```python
from build123d import *

# Parameters (mm, degrees)
F0_R     = 38.1
F0_R_2   = 31.750001
F1_DEPTH = 104.775
F2_R     = 2.4892
F3_DEPTH = 101.6
F4_R     = 2.4892
F5_DEPTH = 101.6


with BuildPart() as f1:
    # F0 (on Front) → F1 (new body, symmetric)
    with BuildSketch(Plane.XZ):
        Circle(F0_R)
        Circle(F0_R_2, mode=Mode.SUBTRACT)
    extrude(amount=F1_DEPTH, both=True)

    # F2 (on Right) → F3 (cut, symmetric)
    with BuildSketch(Plane.YZ):
        with Locations((95.25, 0)):
            Circle(F2_R)
        with Locations((-95.25, 0)):
            Circle(F2_R)
    extrude(amount=F3_DEPTH, both=True, mode=Mode.SUBTRACT)

    # F4 (on Top) → F5 (cut, symmetric)
    with BuildSketch(Plane.XY):
        with Locations((0, 95.25)):
            Circle(F4_R)
        with Locations((0, -95.25)):
            Circle(F4_R)
    extrude(amount=F5_DEPTH, both=True, mode=Mode.SUBTRACT)


solid = f1.part
```
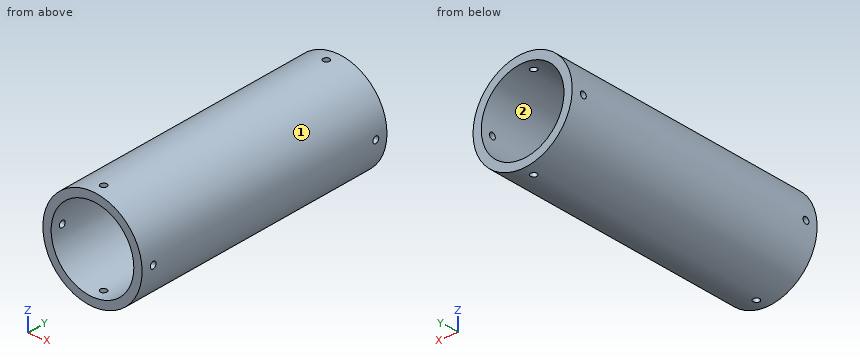
Geometry check sheet. Reference: the model listing, model coordinates, mm. Face numbers are marked on the shaded views. Coordinates: 2 decimals unless noted, no trailing zeros. Write each loop counter-clockwise with the first axis right and the second up, starting at its lowest first coordinate (ties: lowest second). Pieces come first, ordered by that corner, then holes. Notation, with made-up numbers: M 31,-17 L 53,-17 A26 cw 53,14 Z; hole C 86.25,69.25 d6. An arc over 180 degrees is marked long. One line per item, written item: value. Start each with the question number.
(1) Sectioned sample at D-D, the plane z = 16. Enter the section's corners in (x, y) (3 decimals), and give its area (3 significant figures).
(2) Sectioned sample at A-A, the plane x = 0. Enter the section's corners in (y, z) (3 decimals), and give its area (3 significant figures).
(3) Depth check by flat-ended pin: pin 1 (6 mm diameter, centred on y = 34.5, z = -18, fed in from +X); pin 2 (12 mm diameter, centred on x = 8.5, y = -66.5, fed in from -Z); pin 3 (1.5 mm diameter, centred on y = -42.5, z = -16, fed in from -X); pin 4 (1 mm diameter, centred on x = -27.5, z = -10, fed in from -Y). Enter the tip coordinate at first touch or a pass-through.
(4) Sectioned sample at B-B, the plane z = 0. Enter the section's corners in (x, y) (3 decimals), and give its area (3 significant figures).
(5) Scan lines: line 1 along Y through (x, z) = (0, -34.25) (3 decimals); line 2 along Z through (x, y) = (-0.5, 21); line 3 along Z through (x, y) = (-33, -95). Record each from-to range of solid material in increasing order. Write a range as [from, to].
(6) Sectioned sample at C-C, the plane y = -95.25. Enter the section's corners in (x, z), and give its area (3 significant figures).
(7) Release check for a two-part mould opening along Z. For the marked faces 1 and 2 record: released by +Z, released by -Z, zero draft, split by the parting line, or undercut.
Filled sheet:
1. outline: M -34.578,-104.775 L -27.424,-104.775 L -27.424,104.775 L -34.578,104.775 Z; M 27.424,-104.775 L 34.578,-104.775 L 34.578,104.775 L 27.424,104.775 Z
1. area: 3,000 mm²
2. outline: M -104.775,-38.1 L -97.739,-38.1 L -97.739,-31.75 L -104.775,-31.75 Z; M -104.775,31.75 L -97.739,31.75 L -97.739,38.1 L -104.775,38.1 Z; M -92.761,-38.1 L 92.761,-38.1 L 92.761,-31.75 L -92.761,-31.75 Z; M -92.761,31.75 L 92.761,31.75 L 92.761,38.1 L -92.761,38.1 Z; M 97.739,-38.1 L 104.775,-38.1 L 104.775,-31.75 L 97.739,-31.75 Z; M 97.739,31.75 L 104.775,31.75 L 104.775,38.1 L 97.739,38.1 Z
2. area: 2,530 mm²
3. pin 1: x = 35.02
3. pin 2: z = -38.02
3. pin 3: x = -34.91
3. pin 4: through
4. outline: M -38.1,-104.775 L -31.75,-104.775 L -31.75,-97.739 L -38.1,-97.739 Z; M -38.1,-92.761 L -31.75,-92.761 L -31.75,92.761 L -38.1,92.761 Z; M -38.1,97.739 L -31.75,97.739 L -31.75,104.775 L -38.1,104.775 Z; M 31.75,-104.775 L 38.1,-104.775 L 38.1,-97.739 L 31.75,-97.739 Z; M 31.75,-92.761 L 38.1,-92.761 L 38.1,92.761 L 31.75,92.761 Z; M 31.75,97.739 L 38.1,97.739 L 38.1,104.775 L 31.75,104.775 Z
4. area: 2,530 mm²
5. line 1: [-104.775, -97.739], [-92.761, 92.761], [97.739, 104.775]
5. line 2: [-38.1, -31.75], [31.75, 38.1]
5. line 3: [-19.04, -2.48], [2.48, 19.04]
6. outline: M -38.02,-2.49 A38.1 ccw -2.49,-38.02 L -2.49,-31.65 A31.75 cw -31.65,-2.49 Z; M -38.02,2.49 L -31.65,2.49 A31.75 cw -2.49,31.65 L -2.49,38.02 A38.1 ccw Z; M 2.49,-38.02 A38.1 ccw 38.02,-2.49 L 31.65,-2.49 A31.75 cw 2.49,-31.65 Z; M 2.49,31.65 A31.75 cw 31.65,2.49 L 38.02,2.49 A38.1 ccw 2.49,38.02 Z
6. area: 1,270 mm²
7. face 1: split by the parting line
7. face 2: undercut
